Build history of the part. All positions in model axes, mm. Face numbers are marked on the shaded views. A direction names the side the tool comes from. Give positions to 0.01 mm unless a question says otherwise; leave off trailing zeros. Write each loop counter-clockwise with the first axis right and the second up, starting at its lowest first coordinate (ties: lowest second). Pieces come first, ordered by that corner, then holes.
from build123d import *

# Parameters (mm, degrees)
SKETCH1_W                    = 50.8
SKETCH1_H                    = 12.7
BOSS_EXTRUDE1_DEPTH          = 44.45
SKETCH8_W                    = 13.97
SKETCH8_H                    = 19.685
SKETCH8_W_2                  = 22.86
SKETCH8_W_3                  = 38.1
SKETCH8_H_2                  = 15.875
CUT_EXTRUDE1_DEPTH           = 53.74706153
F_8_CLEARANCE_HOLE3_D        = 4.4958
F_8_CLEARANCE_HOLE2_D        = 4.4958
F_1_8_0_18_DOWEL_HOLE1_D     = 4.572
F_1_8_0_18_DOWEL_HOLE1_DEPTH = 7.62
F_1_8_0_18_DOWEL_HOLE1_TIP   = 1.373567375
FILLET1_R                    = 2.54


with BuildPart() as part:
    # Sketch1 → Boss-Extrude1 (new body)
    with BuildSketch(Plane(origin=(0, 0, 0), x_dir=(1, 0, 0), z_dir=(0, 1, 0))):
        Rectangle(SKETCH1_W, SKETCH1_H)
    extrude(amount=BOSS_EXTRUDE1_DEPTH)

    # Sketch8 → Cut-Extrude1 (cut, through all)
    with BuildSketch(Plane.XY.offset(6.35)):
        with Locations((-18.415, 9.8425)):
            Rectangle(SKETCH8_W, SKETCH8_H)
        with Locations((0, 9.8425)):
            Rectangle(SKETCH8_W_2, SKETCH8_H)
        with Locations((0, 36.5125)):
            Rectangle(SKETCH8_W_3, SKETCH8_H_2)
    extrude(amount=-CUT_EXTRUDE1_DEPTH, mode=Mode.SUBTRACT)

    # #8 Clearance Hole3 (through all)
    with Locations(Plane(origin=(25.4, 0, 0), x_dir=(0, 0, -1), z_dir=(1, 0, 0))):
        with Locations((0, 36.451492413)):
            Hole(F_8_CLEARANCE_HOLE3_D / 2)

    # #8 Clearance Hole2 (through all)
    with Locations(Plane(origin=(0, 28.575, 0), x_dir=(1, 0, 0), z_dir=(0, 1, 0))):
        with Locations((0, 0)):
            Hole(F_8_CLEARANCE_HOLE2_D / 2)

    # 1/8 (0.18) Dowel Hole1
    with Locations(Plane.ZY.offset(-11.43)):
        with Locations((0, 6.096)):
            Hole(F_1_8_0_18_DOWEL_HOLE1_D / 2, depth=F_1_8_0_18_DOWEL_HOLE1_DEPTH)
            with Locations((0, 0, -(F_1_8_0_18_DOWEL_HOLE1_DEPTH + F_1_8_0_18_DOWEL_HOLE1_TIP / 2))):  # 118° drill point
                Cone(0, F_1_8_0_18_DOWEL_HOLE1_D / 2, F_1_8_0_18_DOWEL_HOLE1_TIP, mode=Mode.SUBTRACT)

    # Fillet1
    fillet1_edges = [part.edges().sort_by_distance(p)[0] for p in [
        (11.43, 19.685, 0),
        (19.05, 28.575, 0),
        (-19.05, 28.575, 0),
    ]]
    fillet(fillet1_edges, radius=FILLET1_R)


solid = part.part
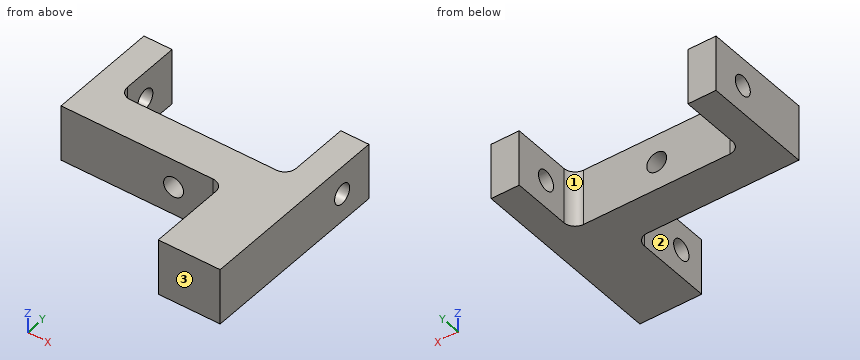
1. Saw through at C-C on y = 23. Give the cut face in (x, z).
2. Saw through at A-A on x = 0. Give the cut face in (y, z) (3 decimals), plus the area to 3 significant figures.
3. Saw through at B-B on z = 3.25. Give the cut face in (x, y) (3 decimals).
4. Drop flat-ended pins along their axis: pin 1 (6 mm diameter, centred on x = 0, z = 0, fed in from -Y) (3 decimals); pin 2 (1 mm diameter, centred on x = -6.5, z = 0.5, fed in from +Y) (3 decimals). Give the stop position or say it passes through.
5. Drill centre lines: line 1 along X through (y, z) = (31, 3.5); line 2 along Y through (x, z) = (22.5, 0); line 3 along Z through (x, y) = (0, 25). Where is each one in solid material? Low to high.
6. 3-axis set-ups, long thin cutter, end or side, ignore diameter. For the marked faces 1, 2 and 3: which of +Z, -Z, +X, -X, +Y, -Y reach the whole face in a straight line?
Outcome:
1. outline: (-25.4, -6.35) - (25.4, -6.35) - (25.4, 6.35) - (-25.4, 6.35) - close; hole circle Ø4.5 at (0, 0)
2. outline: (19.685, -6.35) - (28.575, -6.35) - (28.575, -2.248) - (19.685, -2.248) - close; (19.685, 2.248) - (28.575, 2.248) - (28.575, 6.35) - (19.685, 6.35) - close
2. area: 72.9 mm2
3. outline: (-25.4, 19.685) - (8.89, 19.685) arc R2.54 cw to (11.43, 17.145) - (11.43, 0) - (25.4, 0) - (25.4, 44.45) - (19.05, 44.45) - (19.05, 31.115) arc R2.54 cw to (16.51, 28.575) - (-16.51, 28.575) arc R2.54 cw to (-19.05, 31.115) - (-19.05, 44.45) - (-25.4, 44.45) - close
4. pin 1: stops at y = 19.685
4. pin 2: stops at y = 28.575
5. line 1: x = -25.4 to -19.05, 19.05 to 25.4
5. line 2: y = 0 to 34.2, 38.7 to 44.45
5. line 3: z = -6.35 to -2.25, 2.25 to 6.35
6. face 1: +Z, -Z, +Y
6. face 2: +Z, -Z, -X, -Y
6. face 3: +Z, -Z, +X, -X, -Y
